Geometry: final body of the model. Coordinates: model frame, mm. A direction names the side the tool comes from. Give positions to 0.01 mm unless a question says otherwise; leave off trailing zeros. Loops run counter-clockwise (first coordinate to the right, second up) from the corner with the lowest first, then second, coordinate; pieces in that order, holes last.
1. First-contact query: P1, Ø6, axis at x = -5, z = 10, coming from the +Y side; P2, Ø1.9, axis at x = 0, y = 13.5, coming from the -Z side; P3, Ø1.1, axis at x = 0, y = -10.5, coming from the -Z side; P4, Ø1.6, axis at x = -11.69, y = -6.75, coming from the +Z side. Flat tips, straight axial feed; report the tip coordinate or a pass-through.
2. Section B-B, the plane y = -0.5. Output: boundary loops of the cut face in (x, z).
3. Section D-D, the plane y = -11.5. Output: boundary loops of the cut face in (x, z).
4. Section C-C, the plane y = 10.5. Output: boundary loops of the cut face in (x, z), then the cut area to 3 significant figures.
5. Material intervals for line 1 along Y through (x, z) = (0, 7); line 2 along Y through (x, z) = (14.5, 2.75); line 3 along X through (y, z) = (-1, 7.75), sorted ascending.
6. Draft query along Y for faces 5 (the face through (-9.68, 2.29, 8.34)), 6 (the face through (9.139, 14.334, 2.169)), 7 (the face through (-11.821, -6.164, 3.834)). Return one class per face: +Y half, -Y half, draft (parallel to the pull), parting line (faces both ways), or undercut.
7. Access query for faces 1 (the face through (3, 9.526, 8)), 2 (the face through (7.3, -7.3, 4.4)), 3 (the face through (3.006, 10.933, 1.619)), 4 (the face through (8.288, 4.696, 8.344)). Directions: +Z, -Z, +X, -X, +Y, -Y. A direction counts if a zero-diameter tool reaches every point of the face in a straight line with its end or side. Return the directions, or none.
from build123d import *

# Parameters (mm, degrees)
SKETCH1_R               = 17
BOSS_EXTRUDE1_DEPTH     = 4.4
CAVITY1_OUTLINE_R       = 3.15
CAVITY1_DEPTH           = 3.283595969
CAVITY1_START           = 1.183595969
CAVITY1_2_OUTLINE_R     = 3.15
CAVITY1_2_OUTLINE_R_2   = 1.575
CAVITY1_2_DEPTH         = 2.1
BOSS_EXTRUDE8_DEPTH     = 8
SKETCH2_R               = 0.6
CUT_EXTRUDE1_DEPTH      = 28.051062826
CIRPATTERN1_COUNT       = 6
CUT_EXTRUDE2_START      = -3.283596
SKETCH3_R               = 4.596048158
CUT_EXTRUDE2_DEPTH      = 3.283596
CUT_EXTRUDE3_DEPTH      = 28.051062826
CUT_EXTRUDE3_DEPTH_BACK = 4
SKETCH4_R               = 4
SKETCH6_R               = 1.8
CUT_EXTRUDE4_DEPTH      = 28.051062826


with BuildPart() as part:
    # Sketch1 → Boss-Extrude1 (new body)
    with BuildSketch(Plane.XY):
        Circle(SKETCH1_R)
    extrude(amount=BOSS_EXTRUDE1_DEPTH)

    # Cavity1: read off the stored shape, not the designer's step
    # Cavity1 outline → Cavity1 (cut)
    with BuildSketch(Plane.XY):
        with BuildLine():
            Line((3.9375, 6.819950055), (2.048148228, 15.163776711))
            ThreePointArc((2.048148228, 15.163776711), (0, 16.8), (-2.048148228, 15.163776711))
            Line((-2.048148228, 15.163776711), (-3.9375, 6.819950055))
            Line((-3.9375, 6.819950055), (-12.108141735, 9.355636751))
            ThreePointArc((-12.108141735, 9.355636751), (-14.549226784, 8.4), (-14.156289963, 5.80813996))
            Line((-14.156289963, 5.80813996), (-7.875, 0))
            Line((-7.875, 0), (-14.156289963, -5.80813996))
            ThreePointArc((-14.156289963, -5.80813996), (-14.549226784, -8.4), (-12.108141735, -9.355636751))
            Line((-12.108141735, -9.355636751), (-3.9375, -6.819950055))
            Line((-3.9375, -6.819950055), (-2.048148228, -15.163776711))
            ThreePointArc((-2.048148228, -15.163776711), (0, -16.8), (2.048148228, -15.163776711))
            Line((2.048148228, -15.163776711), (3.9375, -6.819950055))
            Line((3.9375, -6.819950055), (12.108141735, -9.355636751))
            ThreePointArc((12.108141735, -9.355636751), (14.549226784, -8.4), (14.156289963, -5.80813996))
            Line((14.156289963, -5.80813996), (7.875, 0))
            Line((7.875, 0), (14.156289963, 5.80813996))
            ThreePointArc((14.156289963, 5.80813996), (14.549226784, 8.4), (12.108141735, 9.355636751))
            Line((12.108141735, 9.355636751), (3.9375, 6.819950055))
        make_face()
        Circle(CAVITY1_OUTLINE_R, mode=Mode.SUBTRACT)
    extrude(amount=CAVITY1_DEPTH, mode=Mode.SUBTRACT)

    # Cavity1 2 outline → Cavity1 2 (cut)
    with BuildSketch(Plane.XY.offset(CAVITY1_START)):
        Circle(CAVITY1_2_OUTLINE_R)
        Circle(CAVITY1_2_OUTLINE_R_2, mode=Mode.SUBTRACT)
    extrude(amount=CAVITY1_2_DEPTH, mode=Mode.SUBTRACT)

    # Sketch12 → Boss-Extrude8 (add)
    with BuildSketch(Plane.XY.offset(4.4)):
        Polygon((5.5, -9.526279442), (11, 0), (5.5, 9.526279442), (-5.5, 9.526279442), (-11, 0), (-5.5, -9.526279442), align=None)
    extrude(amount=BOSS_EXTRUDE8_DEPTH)

    # Sketch2 → Cut-Extrude1 (cut, through all)
    with BuildSketch(Plane(origin=(0, 0, 0), x_dir=(-1, 0, 0), z_dir=(0, 0, -1))):
        with Locations(Location((0, 13.5, 0), (0, 0, 180))):
            Circle(SKETCH2_R)
        with Locations(Location((0, 10.5, 0), (0, 0, 180))):
            Circle(SKETCH2_R)
        with Locations((0, 7.5)):
            Circle(SKETCH2_R)
    cut_extrude1 = extrude(amount=-CUT_EXTRUDE1_DEPTH, mode=Mode.SUBTRACT)

    # CirPattern1: Cut-Extrude1 ×6 about axis
    cirpattern1_axis = Axis((0, 0, 0), (0, 0, 1))
    for i in range(1, CIRPATTERN1_COUNT):
        add(cut_extrude1.rotate(cirpattern1_axis, i * 360 / CIRPATTERN1_COUNT), mode=Mode.SUBTRACT)

    # Sketch3 → Cut-Extrude2 (cut)
    with BuildSketch(Plane(origin=(0, 0, 0), x_dir=(-1, 0, 0), z_dir=(0, 0, -1)).offset(CUT_EXTRUDE2_START)):
        Circle(SKETCH3_R)
    extrude(amount=CUT_EXTRUDE2_DEPTH, mode=Mode.SUBTRACT)

    # Sketch4 → Cut-Extrude3 (cut, two sides: drawn at the far end of the back side and taken through both)
    with BuildSketch(Plane.XY.offset(-CUT_EXTRUDE3_DEPTH_BACK)):
        Circle(SKETCH4_R)
    extrude(amount=CUT_EXTRUDE3_DEPTH + CUT_EXTRUDE3_DEPTH_BACK, mode=Mode.SUBTRACT)

    # Sketch6 → Cut-Extrude4 (cut, through all)
    with BuildSketch(Plane(origin=(0, 0, 0), x_dir=(-1, 0, 0), z_dir=(0, 0, -1))):
        with Locations((-7.875, 0)):
            Circle(SKETCH6_R)
        with Locations((7.875, 0)):
            Circle(SKETCH6_R)
    extrude(amount=-CUT_EXTRUDE4_DEPTH, mode=Mode.SUBTRACT)

    # Fillet1
    # a fillet whose section is not a circle: 10 mm, written as the material it takes off along each edge
    with BuildSketch(Plane(origin=(-5.5, 9.526279442, 4.4), x_dir=(1, 0, 0), z_dir=(0, 0, 1))) as fillet1_piece_1:
        with BuildLine():
            Bezier((5.773502692, 0), (0, 0), (-2.886751346, -5), weights=[1, 2.333333333, 1])
            Line((-2.886751346, -5), (0, 0))
            Line((0, 0), (5.773502692, 0))
        make_face()
    extrude(amount=22.43375673, mode=Mode.SUBTRACT)


solid = part.part
Answers below:
1. P1: stops at y = 9.47
1. P2: stops at z = 3.28
1. P3: passes through
1. P4: stops at z = 4.4
2. outline: (-16.99, 0) - (-9.6, 0) - (-9.6, 12.4) - (-10.71, 12.4) - (-10.71, 4.4) - (-16.99, 4.4) - close; (-6.15, 3.28) - (-3.97, 3.28) - (-3.97, 12.4) - (-6.15, 12.4) - close; (3.97, 3.28) - (6.15, 3.28) - (6.15, 12.4) - (3.97, 12.4) - close; (9.6, 0) - (16.99, 0) - (16.99, 4.4) - (10.71, 4.4) - (10.71, 12.4) - (9.6, 12.4) - close
3. outline: (-12.52, 0) - (-2.88, 0) - (-2.88, 3.28) - (2.88, 3.28) - (2.88, 0) - (12.52, 0) - (12.52, 4.4) - (-12.52, 4.4) - close
4. outline: (-13.37, 0) - (-3.1, 0) - (-3.1, 3.28) - (-0.6, 3.28) - (-0.6, 4.4) - (-13.37, 4.4) - close; (0.6, 3.28) - (3.1, 3.28) - (3.1, 0) - (13.37, 0) - (13.37, 4.4) - (0.6, 4.4) - close
4. area: 95.9 mm2
5. line 1: y = -9.53 to -8.1, -6.9 to -4, 4 to 6.9, 8.1 to 9.53
5. line 2: y = -8.87 to -8.48, -6.22 to 6.22, 8.48 to 8.87
5. line 3: x = -10.42 to -9.37, -6.38 to -3.87, 3.87 to 6.38, 9.37 to 10.42
6. face 5: +Y half
6. face 6: parting line
6. face 7: undercut
7. face 1: +Z, +X, -X, +Y
7. face 2: +Z
7. face 3: -Z
7. face 4: +Z, +X, +Y
